Input: part model. Units: mm. Frame: model coordinates. Give positions to 0.01 mm unless a question says otherwise; leave off trailing zeros. Loops run counter-clockwise (first coordinate to the right, second up) from the corner with the lowest first, then second, coordinate; pieces in that order, holes last. Notation, with made-up numbers: (58, 52) -> (71, 52) arc R36 ccw to (71, 87) -> close; hole circle Ø2 at (47.5, -16). An arc over 180 degrees is marked (long way). Answer as a JSON object with one key per item and string values.
```python
from build123d import *

# Parameters (mm, degrees)
F0_W     = 75
F0_H     = 25
F1_DEPTH = 2
F2_R     = 0.45
F3_DEPTH = 13.5


with BuildPart() as f1:
    # F0 (on Top) → F1 (new body, symmetric)
    with BuildSketch(Plane.XY):
        Rectangle(F0_W, F0_H)
    extrude(amount=F1_DEPTH, both=True)

    # F2 (on Front) → F3 (join, symmetric)
    with BuildSketch(Plane.XZ):
        Circle(F2_R)
        with Locations((-5.9, 0)):
            Circle(F2_R)
        with Locations((-11.8, 0)):
            Circle(F2_R)
        with Locations((-17.7, 0)):
            Circle(F2_R)
        with Locations((-23.6, 0)):
            Circle(F2_R)
        with Locations((-29.5, 0)):
            Circle(F2_R)
        with Locations((-35.4, 0)):
            Circle(F2_R)
        with Locations((5.9, 0)):
            Circle(F2_R)
        with Locations((11.8, 0)):
            Circle(F2_R)
        with Locations((17.7, 0)):
            Circle(F2_R)
        with Locations((23.6, 0)):
            Circle(F2_R)
        with Locations((29.5, 0)):
            Circle(F2_R)
        with Locations((35.4, 0)):
            Circle(F2_R)
    extrude(amount=F3_DEPTH, both=True)


solid = f1.part
```
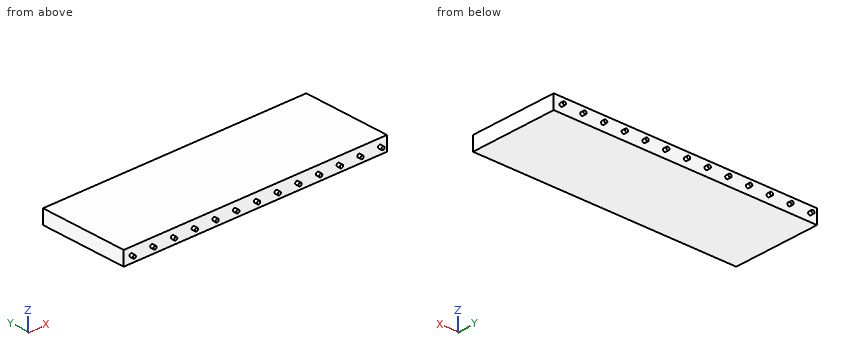
Q1. Ray query, line 1 along Y through (x, z) = (27, 0.2). Return the intervals inside material, ascending.
Evaluation:
{"line 1": "y = -12.5 to 12.5"}
Q2. Pin query (flat end, axial travel): pin 1 (1 mm diameter, centred on x = -8, z = 1.5, fed in from +Y); pin 2 (1.5 mm diameter, centred on x = 11.5, z = -0.5, fed in from -Y). Return the tip coordinate at first contact, or that it passes through.
Evaluation:
{"pin 1": "stops at y = 12.5", "pin 2": "stops at y = -13.5"}
Q3. Section A-A, the plane z = 1.4. Return the cut outline in (x, y).
Evaluation:
{"outline": "(-37.5, -12.5) -> (37.5, -12.5) -> (37.5, 12.5) -> (-37.5, 12.5) -> close"}
Q4. Section B-B, the plane x = -32. Return the cut outline in (y, z).
Evaluation:
{"outline": "(-12.5, -2) -> (12.5, -2) -> (12.5, 2) -> (-12.5, 2) -> close"}
